The listing builds one solid part. Answer for the finished solid, in the listing's coordinates (mm). A direction names the side the tool comes from. Coordinates: 2 decimals unless noted, no trailing zeros. Loops run counter-clockwise (first coordinate to the right, second up) from the corner with the lowest first, then second, coordinate; pieces in that order, holes last. Notation, with made-up numbers: M -3,7 L 43,7 A23 cw 43,29 Z; hole C 49,24 d7. An arc over 180 degrees is marked long. Return JSON: item names as keys, results as strings. Group by question number.
1. Given P1, Ø8, axis at x = 7.5, y = 146.5, coming from the +Z side, flat-ended and moving along its own axis, determine where the tip first touches the part or whether it passes through.
2. The mould has two halves that part along X. Classify faces 1 (the face through (39.527, 40.359, 1.972)), 2 (the face through (67, 185, 5)), 3 (the face through (0, 91, 5)): pulls with the +X half, pulls with the -X half, needs draft (parallel to the pull), parting line crosses it, or undercut.
3. Section B-B (x = 52) is taken. Write down the section's boundary in (y, z).
4. Straight lines are drawn through the part: L1, parallel to Y at x = 7.5, z = 8.3; L2, parallel to Y at x = 127.5, z = 1.6; L3, parallel to X at y = 178.5, z = 1.5. For each, find the intervals that lie inside material, in ascending order. Write a range as from..to.
5. Section A-A (y = 54) is taken. Write down the section's boundary in (x, z).
6. Which of the six approach directions +Z, -Z, +X, -X, +Y, -Y give full straight-line access (tool end or side, diameter ignored) to faces 4 (the face through (100.247, 38.621, 1.972)), 5 (the face through (9, 181, 4))?
7. Section C-C (z = 8.25) is taken. Count the separate pieces of the cut face and the enclosed holes in it, then the cut area to 3 significant figures.
```python
from build123d import *

# Parameters (mm, degrees)
SZKIC1_W                                             = 135
SZKIC1_H                                             = 185
DODANIE_WYCI_GNI_CIE1_DEPTH                          = 10
POG_BIENIE_WALCOWE_POD_M5_WKR_T_DO_CZ_CI_D           = 5.5
POG_BIENIE_WALCOWE_POD_M5_WKR_T_DO_CZ_CI_CBORE_D     = 9
POG_BIENIE_WALCOWE_POD_M5_WKR_T_DO_CZ_CI_CBORE_DEPTH = 6
SZKIC5_R                                             = 2.75
WYTNIJ_WYCI_GNI_CIE1_DEPTH                           = 230.237867727


with BuildPart() as part:
    # Szkic1 → Dodanie-wyciągnięcie1 (new body)
    with BuildSketch(Plane.XY):
        with Locations((67.5, 92.5)):
            Rectangle(SZKIC1_W, SZKIC1_H)
    extrude(amount=DODANIE_WYCI_GNI_CIE1_DEPTH)

    # Pogłębienie walcowe pod M5 Wkręt do części metalowych z łbem sześciokątnym1 (through all)
    with Locations(Plane.XY.offset(10)):
        with Locations((7.5, 178.5), (37.5, 178.5), (37.5, 146.5), (7.5, 146.5), (7.5, 38.5), (37.5, 38.5), (7.5, 6.5), (37.5, 6.5), (97.5, 6.5), (127.5, 6.5), (97.5, 38.5), (127.5, 38.5), (127.5, 146.5), (97.5, 146.5), (97.5, 178.5), (127.5, 178.5)):
            CounterBoreHole(POG_BIENIE_WALCOWE_POD_M5_WKR_T_DO_CZ_CI_D / 2, POG_BIENIE_WALCOWE_POD_M5_WKR_T_DO_CZ_CI_CBORE_D / 2, POG_BIENIE_WALCOWE_POD_M5_WKR_T_DO_CZ_CI_CBORE_DEPTH)

    # Szkic5 → Wytnij-wyciągnięcie1 (cut, through all)
    with BuildSketch(Plane.XY.offset(10)):
        with Locations((22, 54)):
            Circle(SZKIC5_R)
        with Locations((52, 23)):
            Circle(SZKIC5_R)
        with Locations((85, 23)):
            Circle(SZKIC5_R)
        with Locations((115, 54)):
            Circle(SZKIC5_R)
        with Locations(Location((52, 162, 0), (0, 0, 180))):
            Circle(SZKIC5_R)
        with Locations(Location((22, 131, 0), (0, 0, 180))):
            Circle(SZKIC5_R)
        with Locations(Location((115, 131, 0), (0, 0, 180))):
            Circle(SZKIC5_R)
        with Locations(Location((85, 162, 0), (0, 0, 180))):
            Circle(SZKIC5_R)
    extrude(amount=-WYTNIJ_WYCI_GNI_CIE1_DEPTH, mode=Mode.SUBTRACT)


solid = part.part
```
Worked out:
{
 "1": {"P1": "z = 4"},
 "2": {"face 1": "undercut", "face 2": "needs draft", "face 3": "pulls with the -X half"},
 "3": {"outline": "M 0,0 L 20.25,0 L 20.25,10 L 0,10 Z; M 25.75,0 L 159.25,0 L 159.25,10 L 25.75,10 Z; M 164.75,0 L 185,0 L 185,10 L 164.75,10 Z"},
 "4": {"L1": "0..2, 11..34, 43..142, 151..174, 183..185", "L2": "0..3.75, 9.25..35.75, 41.25..143.75, 149.25..175.75, 181.25..185", "L3": "0..4.75, 10.25..34.75, 40.25..94.75, 100.25..124.75, 130.25..135"},
 "5": {"outline": "M 0,0 L 19.25,0 L 19.25,10 L 0,10 Z; M 24.75,0 L 112.25,0 L 112.25,10 L 24.75,10 Z; M 117.75,0 L 135,0 L 135,10 L 117.75,10 Z"},
 "6": {"face 4": "+Z, -Z", "face 5": "+Z"},
 "7": {"separate pieces": "1", "enclosed holes": "24", "area": "23,800 mm^2"}
}
